```python
from build123d import *

# Parameters (mm, degrees)
F0_R     = 11
F0_R_2   = 6.5
F1_DEPTH = 1.5
F0_R_3   = 1.5
F2_DEPTH = 2.5
F3_R     = 0.49999


# Not quite as in the source:
# - a fillet or chamfer is up to 0.001 mm smaller than in the source, because OpenCascade refuses the exact size


with BuildPart() as f1:
    # F0 (on Top) → F1 (new body)
    with BuildSketch(Plane.XY):
        Circle(F0_R)
        Circle(F0_R_2, mode=Mode.SUBTRACT)
    extrude(amount=F1_DEPTH)

    # F0 (on Top) → F2 (join)
    with BuildSketch(Plane.XY):
        Circle(F0_R_2)
        with Locations((-2, 0)):
            Circle(F0_R_3, mode=Mode.SUBTRACT)
        with Locations((2, 0)):
            Circle(F0_R_3, mode=Mode.SUBTRACT)
    extrude(amount=F2_DEPTH)

    # F3 (radius 0.5 in the source; OpenCascade refuses exactly that, so slightly less here)
    f3_edges = [f1.edges().sort_by_distance(p)[0] for p in [
        (-11, 0, 1.5),
        (-6.5, 0, 1.5),
        (-6.5, 0, 2.5),
        (0.5, 0, 2.5),
        (-3.5, 0, 2.5),
    ]]
    fillet(f3_edges, radius=F3_R)


solid = f1.part
```
CAD build for the part. Positions are in the model's coordinates, mm. Give positions to 0.01 mm unless a question says otherwise; leave off trailing zeros. Return JSON: item names as keys, results as strings. Group by question number.
(1) Drill centre lines: L1, parallel to X at y = 1, z = 0.65; L2, parallel to Y at x = 2, z = 1.65; L3, parallel to Z at x = 5, y = 5. Where is each one in solid material? Low to high. Write a range as [from, to].
(2) Band-saw the part on A-A (y = 0). State how many separate pieces and enclosed holes the cut face has, and give its area (3 significant figures).
(3) Flat gauge pins, fed straight in: pin 1 Ø8 at (x, y) = (8.5, 4.5) entering from +Z; pin 2 Ø1.8 at (x, y) = (2, 0) entering from -Z. Where does each tip first touch, or does it go through?
(4) Mould opens along Y. For faces 1 (the face through (-2.38, -10.74, 0.49)), 2 (the face through (2, -7, 1.5)), 3 (the face through (0.5, 0.07, 0.99)) say: pulls with the +Y half, pulls with the -Y half, needs draft (parallel to the pull), parting line crosses it, or undercut.
Entries:
{
 "1": {"L1": "x = [-10.95, -3.12], [-0.88, 0.88], [3.12, 10.95]", "L2": "y = [-6.33, -1.5], [1.5, 6.33]", "L3": "z = [0, 1.5]"},
 "2": {"separate pieces": "3", "enclosed holes": "0", "area": "30.7 mm^2"},
 "3": {"pin 1": "stops at z = 2.5", "pin 2": "passes through"},
 "4": {"face 1": "parting line crosses it", "face 2": "needs draft", "face 3": "undercut"}
}
